Input: part model. Units: mm. Frame: model coordinates. Face numbers are marked on the shaded views. Coordinates: 2 decimals unless noted, no trailing zeros. Loops run counter-clockwise (first coordinate to the right, second up) from the corner with the lowest first, then second, coordinate; pieces in that order, holes last.
Item 1: Section C-C on z = 3.2. Return loops of the section in (x, y), and give its area (3 significant figures).
Item 2: Contact query for flat-ended pins moving along their axis: P1, Ø4, axis at x = -23.57, y = 23.57, coming from the -Z side (3 decimals); P2, Ø1.5, axis at x = 8, y = 9, coming from the +Z side; P3, Ø1, axis at x = -7, y = 2.5, coming from the -Z side. Output: stop coordinate, or through.
Item 3: Ray query, line 1 along Y through (x, z) = (23.57, 1); line 2 along X through (y, z) = (23, 0.85); line 3 along Y through (x, z) = (0, 0.5). Return the intervals inside material, ascending.
Item 4: Section D-D on x = 22. Return loops of the section in (y, z).
Item 5: Section A-A on y = 0. Return loops of the section in (x, z).
Item 6: Pull-direction query (X, two-part tool) for the marked faces 1 and 2; classes: released by +X, released by -X, zero draft, split by the parting line, or undercut.
```python
from build123d import *

# Parameters (mm, degrees)
SKIZZE1_W                       = 57
SKIZZE1_H                       = 57
AUFSATZ_LINEAR_AUSTRAGEN1_DEPTH = 4
F_5_0_5_DURCHMESSER_BOHRUNG2_D  = 5
VERRUNDUNG1_R                   = 5
SKIZZE6_R                       = 19.1
SCHNITT_LINEAR_AUSTRAGEN1_DEPTH = 2
F_8_0_8_DURCHMESSER_BOHRUNG1_D  = 8


with BuildPart() as part:
    # Skizze1 → Aufsatz-Linear austragen1 (new body)
    with BuildSketch(Plane.XY):
        Rectangle(SKIZZE1_W, SKIZZE1_H)
    extrude(amount=AUFSATZ_LINEAR_AUSTRAGEN1_DEPTH)

    # Ø5.0 (5) Durchmesser Bohrung2 (through all)
    with Locations(Plane.XY.offset(4)):
        with Locations((-23.57, 23.57), (23.57, 23.57), (23.57, -23.57), (-23.57, -23.57)):
            Hole(F_5_0_5_DURCHMESSER_BOHRUNG2_D / 2)

    # Verrundung1
    verrundung1_edges = [part.edges().sort_by_distance(p)[0] for p in [
        (28.5, -28.5, 2),
        (-28.5, -28.5, 2),
        (-28.5, 28.5, 2),
        (28.5, 28.5, 2),
    ]]
    fillet(verrundung1_edges, radius=VERRUNDUNG1_R)

    # Skizze6 → Schnitt-Linear austragen1 (cut)
    with BuildSketch(Plane.XY.offset(4)):
        Circle(SKIZZE6_R)
    extrude(amount=-SCHNITT_LINEAR_AUSTRAGEN1_DEPTH, mode=Mode.SUBTRACT)

    # Ø8.0 (8) Durchmesser Bohrung1 (through all)
    with Locations(Plane.XY.offset(2)):
        with Locations((0, 0)):
            Hole(F_8_0_8_DURCHMESSER_BOHRUNG1_D / 2)


solid = part.part
```
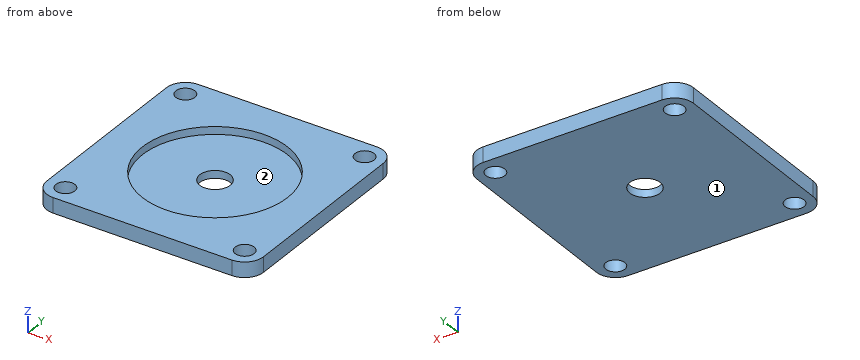
Results found:
1. outline: (-28.5, -23.5) arc R5 ccw to (-23.5, -28.5) - (23.5, -28.5) arc R5 ccw to (28.5, -23.5) - (28.5, 23.5) arc R5 ccw to (23.5, 28.5) - (-23.5, 28.5) arc R5 ccw to (-28.5, 23.5) - close; hole circle Ø5 at (-23.57, -23.57); hole circle Ø5 at (-23.57, 23.57); hole circle Ø38.2 at (0, 0); hole circle Ø5 at (23.57, -23.57); hole circle Ø5 at (23.57, 23.57)
1. area: 2,000 mm2
2. P1: passes through
2. P2: stops at z = 2
2. P3: stops at z = 0
3. line 1: y = -28.5 to -26.07, -21.07 to 21.07, 26.07 to 28.5
3. line 2: x = -28.5 to -26, -21.14 to 21.14, 26 to 28.5
3. line 3: y = -28.5 to -4, 4 to 28.5
4. outline: (-28.5, 0) - (-25.52, 0) - (-25.52, 4) - (-28.5, 4) - close; (-21.62, 0) - (21.62, 0) - (21.62, 4) - (-21.62, 4) - close; (25.52, 0) - (28.5, 0) - (28.5, 4) - (25.52, 4) - close
5. outline: (-28.5, 0) - (-4, 0) - (-4, 2) - (-19.1, 2) - (-19.1, 4) - (-28.5, 4) - close; (4, 0) - (28.5, 0) - (28.5, 4) - (19.1, 4) - (19.1, 2) - (4, 2) - close
6. face 1: zero draft
6. face 2: undercut
